For this review, use the dimensioned drawing (mm, ordinates from the lowest corner) and the shaded views. Coordinates: 2 decimals unless noted, no trailing zeros. Loops run counter-clockwise (first coordinate to the right, second up) from the corner with the lowest first, then second, coordinate; pieces in that order, holes last. Notation, with made-up numbers: M 69,-23 L 84,-23 A7 ccw 84,-14 Z; hole C -11,52.25 d1. An arc over 180 degrees is marked long. Use CSV: the item, a comma, the result in double quotes. Start each with the question number.
1. Add section A-A, the plane x = 32.5. Write out the cut boundary in (y, z) (1 decimal).
2. Add section C-C, the plane z = 27.5. Write out the cut boundary in (x, y) (1 decimal).
3. For L1, parallel to Z at x = 5.5, y = 0.3 (1 decimal); L2, parallel to Z at x = 31, y = 1 (1 decimal); L3, parallel to X at y = 1, z = 6.5, list the stretches that pass through material, from the lowest coordinate up.
4. Add section D-D, the plane x = 58.5. Write out the cut boundary in (y, z) (1 decimal).
5. Clearance check with flat-ended pins moving along their axes: P1, Ø0.8, axis at y = 1, z = 40.5, coming from the -X side; P2, Ø1.5, axis at x = 56, z = 51.5, coming from the -Y side. State where each tip first meets the part, or that it passes through.
6. Add section B-B, the plane y = 0.75. State how many separate pieces and enclosed holes the cut face has, then the cut area to 3 significant figures.
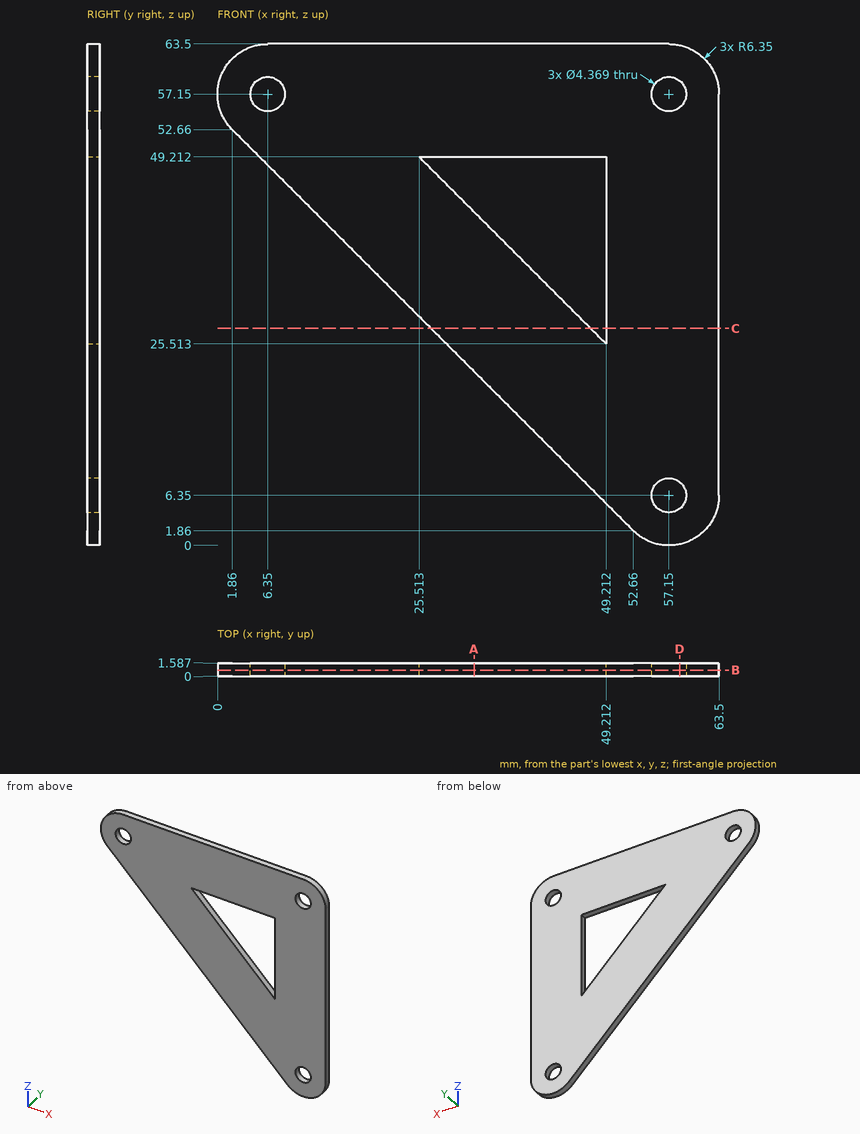
Computed:
1,outline,"M 0,22 L 1.6,22 L 1.6,42.2 L 0,42.2 Z; M 0,49.2 L 1.6,49.2 L 1.6,63.5 L 0,63.5 Z"
2,outline,"M 27,0 L 47.2,0 L 47.2,1.6 L 27,1.6 Z; M 49.2,0 L 63.5,0 L 63.5,1.6 L 49.2,1.6 Z"
3,L1,"z = 49 to 55.1, 59.2 to 63.4"
3,L2,"z = 23.5 to 43.7, 49.2 to 63.5"
3,L3,"x = 48.02 to 54.97, 59.33 to 63.5"
4,outline,"M 0,0.1 L 1.6,0.1 L 1.6,4.6 L 0,4.6 Z; M 0,8.1 L 1.6,8.1 L 1.6,55.4 L 0,55.4 Z; M 0,58.9 L 1.6,58.9 L 1.6,63.4 L 0,63.4 Z"
5,P1,"stops at x = 13.62"
5,P2,"stops at y = 0"
6,separate pieces,"1"
6,enclosed holes,"4"
6,area,"2,190 mm^2"
